```python
from build123d import *

# Parameters (mm, degrees)
BOSS_EXTRUDE1_DEPTH = 20
SKETCH2_R           = 1.75
CUT_EXTRUDE1_DEPTH  = 3.5
SKETCH4_W           = 5.5
SKETCH4_H           = 10
BOSS_EXTRUDE2_DEPTH = 8.75
SKETCH5_R           = 0.875
CUT_EXTRUDE2_DEPTH  = 10
SKETCH6_W           = 3.5
SKETCH6_H           = 6
BOSS_EXTRUDE3_DEPTH = 5
FILLET1_R           = 1
SKETCH8_W           = 6.5
SKETCH8_H           = 3
CUT_EXTRUDE3_DEPTH  = 30
CHAMFER1_SIZE       = 1
SKETCH10_W          = 2
SKETCH10_H          = 10.5
BOSS_EXTRUDE5_DEPTH = 20
SKETCH11_W          = 2
SKETCH11_H          = 20
BOSS_EXTRUDE6_DEPTH = 5
SKETCH12_W          = 7.625
SKETCH12_H          = 20
BOSS_EXTRUDE7_DEPTH = 2
FILLET2_R           = 2


with BuildPart() as part:
    # Sketch1 → Boss-Extrude1 (new body)
    with BuildSketch(Plane.XY):
        Polygon((-16.75, 0), (16.75, 0), (16.75, -10.5), (5, -10.5), (5, -5.5), (5, -3.5), (0.5, -3.5), (0.5, -5.5), (-11.25, -5.5), (-11.25, -10.5), (-16.75, -10.5), align=None)
    extrude(amount=BOSS_EXTRUDE1_DEPTH)

    # Sketch2 → Cut-Extrude1 (cut)
    with BuildSketch(Plane.XZ.offset(3.5)):
        with Locations((2.75, 15)):
            Circle(SKETCH2_R)
        with Locations((2.75, 5)):
            Circle(SKETCH2_R)
    extrude(amount=-CUT_EXTRUDE1_DEPTH, mode=Mode.SUBTRACT)

    # Sketch4 → Boss-Extrude2 (add)
    with BuildSketch(Plane.XZ.offset(10.5)):
        with Locations((-14, 10)):
            Rectangle(SKETCH4_W, SKETCH4_H)
    extrude(amount=BOSS_EXTRUDE2_DEPTH)

    # Sketch5 → Cut-Extrude2 (cut)
    with BuildSketch(Plane.XZ.offset(19.25)):
        with Locations((-14, 10)):
            Circle(SKETCH5_R)
    extrude(amount=-CUT_EXTRUDE2_DEPTH, mode=Mode.SUBTRACT)

    # Sketch6 → Boss-Extrude3 (add, symmetric)
    with BuildSketch(Plane.XY.offset(10)):
        with Locations((10.875, -13.5)):
            Rectangle(SKETCH6_W, SKETCH6_H)
    extrude(amount=BOSS_EXTRUDE3_DEPTH, both=True)

    # Fillet1
    fillet1_edges = [part.edges().sort_by_distance(p)[0] for p in [
        (-14, -10.5, 5),
        (-14, -10.5, 15),
        (10.875, -10.5, 5),
        (10.875, -10.5, 15),
    ]]
    fillet(fillet1_edges, radius=FILLET1_R)

    # Sketch8 → Cut-Extrude3 (cut)
    with BuildSketch(Plane.XY.offset(20)):
        with Locations((2.75, -4)):
            Rectangle(SKETCH8_W, SKETCH8_H)
    extrude(amount=-CUT_EXTRUDE3_DEPTH, mode=Mode.SUBTRACT)

    # Chamfer1
    chamfer1_edges = [part.edges().sort_by_distance(p)[0] for p in [
        (5, -5.5, 10),
    ]]
    chamfer(chamfer1_edges, length=CHAMFER1_SIZE - 0.0001)  # a hair under: the kernel refuses the full size

    # Sketch10 → Boss-Extrude5 (add)
    with BuildSketch(Plane.XY.offset(20)):
        with Locations((-17.75, -5.25)):
            Rectangle(SKETCH10_W, SKETCH10_H)
    extrude(amount=-BOSS_EXTRUDE5_DEPTH)

    # Sketch11 → Boss-Extrude6 (add)
    with BuildSketch(Plane.XZ.offset(10.5)):
        with Locations((-10.25, 10)):
            Rectangle(SKETCH11_W, SKETCH11_H)
    extrude(amount=-BOSS_EXTRUDE6_DEPTH)

    # Sketch12 → Boss-Extrude7 (add)
    with BuildSketch(Plane.XZ.offset(16.5)):
        with Locations((12.9375, 10)):
            Rectangle(SKETCH12_W, SKETCH12_H)
    extrude(amount=BOSS_EXTRUDE7_DEPTH)

    # Fillet2
    fillet2_edges = [part.edges().sort_by_distance(p)[0] for p in [
        (10.875, -16.5, 5),
        (10.875, -16.5, 15),
    ]]
    fillet(fillet2_edges, radius=FILLET2_R)


solid = part.part
```
Could you check a few things on this model? Use its own coordinates, in mm. A direction names the side the tool comes from. Coordinates: 2 decimals unless noted, no trailing zeros. Order: outer loops, then holes, each group sorted by start corner. A loop starts at its lowest first (then second) coordinate and runs counter-clockwise, first axis right, second up. Notation, with made-up numbers: M -30,-36.5 L 0,-36.5 A11 ccw 0,-26.5 Z; hole C -38,33.25 d11. An arc over 180 degrees is marked long. Use a Markdown table: item, result. Add a question column.
Q1. We'd pull the mould along X, two halves only. Please class faces 5 (the flat face through (-5, -5.5, 10)), 6 (the flat face through (-14.04, -19.25, 8.96)): pulls with the +X half, pulls with the -X half, needs draft (parallel to the pull), parting line crosses it, or undercut.
Q2. If I drill on L1, parallel to Z at x = 2.75, y = -1.95; L2, parallel to X at y = -8.75, z = 16.75; L3, parallel to X at y = -4, z = 17.75, over which ranges is the centre line in solid material (lowest first)?
Q3. I want a section at C-C on y = -7.5. List the corners of the cut face in (x, z) for me, then the cut area to 3 significant figures.
Q4. Which directions (+Z, -Z, +X, -X, +Y, -Y) give clear straight access to the entire face, cutting with the end or side of a thin tool? Please do faces 1 (the cylindrical face through (10.9, -10.785, 4.699)), 2 (the flat face through (-9.25, -8, 10)), 3 (the flat face through (-14, -15, 15)), 4 (the flat face through (-17, -10.5, 10)).
Q5. I'm going to push flat-ended pins straight in: pin 1 (4 mm diameter, centred on x = 12, z = 13.5, fed in from -Y); pin 2 (0.9 mm diameter, centred on x = -14, z = 10, fed in from -Y); pin 3 (3 mm diameter, centred on x = -14.5, y = -16, fed in from -Z). Where does each tip first touch, or does it pass through?
Q6. I want a section at B-B on x = 2.75. List the corners of the cut face in (y, z) for me, then the cut area to 3 significant figures.
Q7. I want a section at A-A on y = -13.75. List the corners of the cut face in (x, z) for me (3 decimals), then the cut area to 3 significant figures.
Checked values:
| question | item | result |
|---|---|---|
| 1 | face 5 | undercut |
| 1 | face 6 | needs draft |
| 2 | L1 | 0 to 3.25, 6.75 to 13.25, 16.75 to 20 |
| 2 | L2 | -18.75 to -9.25, 5 to 16.75 |
| 2 | L3 | -18.75 to -0.5, 6 to 16.75 |
| 3 | outline | M -18.75,0 L -9.25,0 L -9.25,20 L -18.75,20 Z; M 5,0 L 16.75,0 L 16.75,20 L 5,20 Z |
| 3 | area | 425 mm² |
| 4 | face 1 | -Z, +X, -X |
| 4 | face 2 | +Z, -Z, -Y |
| 4 | face 3 | +Z, -X, -Y |
| 4 | face 4 | -Y |
| 5 | pin 1 | y = -18.5 |
| 5 | pin 2 | y = -9.25 |
| 5 | pin 3 | z = 5 |
| 6 | outline | M -2.5,0 L 0,0 L 0,3.25 L -2.5,3.25 Z; M -2.5,6.75 L 0,6.75 L 0,13.25 L -2.5,13.25 Z; M -2.5,16.75 L 0,16.75 L 0,20 L -2.5,20 Z |
| 6 | area | 32.5 mm² |
| 7 | outline | M -16.75,5 L -11.25,5 L -11.25,15 L -16.75,15 Z; M 9.125,5 L 12.625,5 L 12.625,15 L 9.125,15 Z; hole C -14,10 d1.75 |
| 7 | area | 87.6 mm² |
